```python
from build123d import *

# Parameters (mm, degrees)
F1_R     = 1.5
F1_R_2   = 4
F2_DEPTH = 37.5
F3_DEPTH = 3
F4_DEPTH = 10


with BuildPart() as f2:
    # F1 (on Front) → F2 (new body)
    with BuildSketch(Plane.XZ):
        with BuildLine():
            ThreePointArc((100, 102), (100.585786, 100.585786), (102, 100))
            Line((102, 100), (139, 100))
            ThreePointArc((139, 100), (140.414214, 100.585786), (141, 102))
            Line((141, 102), (141, 139))
            ThreePointArc((141, 139), (140.414214, 140.414214), (139, 141))
            Line((139, 141), (102, 141))
            ThreePointArc((102, 141), (100.585786, 140.414214), (100, 139))
            Line((100, 139), (100, 102))
        make_face()
        with Locations((104.75, 104.75)):
            Circle(F1_R, mode=Mode.SUBTRACT)
        with Locations((136.25, 104.75)):
            Circle(F1_R, mode=Mode.SUBTRACT)
        with Locations((104.75, 136.25)):
            Circle(F1_R, mode=Mode.SUBTRACT)
        with Locations((120.5, 120.5)):
            Circle(F1_R_2, mode=Mode.SUBTRACT)
        with Locations((136.25, 136.25)):
            Circle(F1_R, mode=Mode.SUBTRACT)
        with Locations((104.75, 136.25)):
            Circle(F1_R)
        with Locations((136.25, 136.25)):
            Circle(F1_R)
        with Locations((120.5, 120.5)):
            Circle(F1_R_2)
        with Locations((136.25, 104.75)):
            Circle(F1_R)
        with Locations((104.75, 104.75)):
            Circle(F1_R)
    extrude(amount=F2_DEPTH)

    # F1 (on Front) → F3 (cut)
    with BuildSketch(Plane.XZ):
        with Locations((136.25, 104.75)):
            Circle(F1_R)
        with Locations((104.75, 104.75)):
            Circle(F1_R)
        with Locations((136.25, 136.25)):
            Circle(F1_R)
        with Locations((104.75, 136.25)):
            Circle(F1_R)
    extrude(amount=F3_DEPTH, mode=Mode.SUBTRACT)

    # F1 (on Front) → F4 (join)
    with BuildSketch(Plane.XZ):
        with Locations((120.5, 120.5)):
            Circle(F1_R_2)
    extrude(amount=-F4_DEPTH)


solid = f2.part
```
Geometry check sheet. Reference: the model listing, model coordinates, mm. A direction names the side the tool comes from. Coordinates: 2 decimals unless noted, no trailing zeros. Order: outer loops, then holes, each group sorted by start corner. A loop starts at its lowest first (then second) coordinate and runs counter-clockwise, first axis right, second up. Notation, with made-up numbers: M 76,43.5 L 114,43.5 A9 cw 114,56.5 Z; hole C 70,-5.75 d11. An arc over 180 degrees is marked long. Answer as a JSON object with one key per item and string values.
Q1. Tool access check on faces 1 (the cylindrical face through (104.555, -1.479, 137.737)), 2 (the flat face through (141, -18, 120)). Record the directions out of +Z, -Z, +X, -X, +Y, -Y that give a thin tool (end or side, any length) a straight path to the whole face; none if there is none.
Results are:
{"face 1": "+Y", "face 2": "+Z, -Z, +X, +Y, -Y"}
Q2. Cross-section at C-C on x = 120.5. Record the cut outline in (y, z), and give its area (3 significant figures).
Results are:
{"outline": "M -37.5,100 L 0,100 L 0,116.5 L 10,116.5 L 10,124.5 L 0,124.5 L 0,141 L -37.5,141 Z", "area": "1,620 mm²"}
Q3. Cross-section at D-D on y = 4. Record the cut outline in (x, z), and give its area (3 significant figures).
Results are:
{"outline": "C 120.5,120.5 d8", "area": "50.3 mm²"}
Q4. Release check for a two-part mould opening along Z. For faces 3 (the cylindrical face through (104.555, -1.479, 106.237)), 4 (the cylindrical face through (140.43, -18.49, 140.4)), 5 (the flat face through (105, -3, 136)), 6 (the flat face through (120, -37.5, 121)) record: released by +Z, released by -Z, zero draft, split by the parting line, or undercut.
Results are:
{"face 3": "undercut", "face 4": "released by +Z", "face 5": "undercut", "face 6": "zero draft"}
Q5. Cross-section at B-B on x = 104.75. Record the cut outline in (y, z).
Results are:
{"outline": "M -37.5,100 L 0,100 L 0,103.25 L -3,103.25 L -3,106.25 L 0,106.25 L 0,134.75 L -3,134.75 L -3,137.75 L 0,137.75 L 0,141 L -37.5,141 Z"}
Q6. Depth check by flat-ended pin: pin 1 Ø0.9 at (x, z) = (104.5, 136) entering from +Y; pin 2 Ø4 at (x, z) = (123.5, 108) entering from +Y; pin 3 Ø6 at (y, z) = (3.5, 116.5) entering from -X. Enter the tip coordinate at first touch or a pass-through.
Results are:
{"pin 1": "stops at y = -3", "pin 2": "stops at y = 0", "pin 3": "stops at x = 116.63"}
Q7. Cross-section at A-A on z = 136.25. Record the cut outline in (x, y), and give its area (3 significant figures).
Results are:
{"outline": "M 100,-37.5 L 141,-37.5 L 141,0 L 137.75,0 L 137.75,-3 L 134.75,-3 L 134.75,0 L 106.25,0 L 106.25,-3 L 103.25,-3 L 103.25,0 L 100,0 Z", "area": "1,520 mm²"}
Q8. Scan lines: line 1 (X direction, y = -1.05, z = 136.25); line 2 (Z direction, x = 104, y = -1). Record each from-to range of solid material in increasing order.
Results are:
{"line 1": "x = 100 to 103.25, 106.25 to 134.75, 137.75 to 141", "line 2": "z = 100 to 103.45, 106.05 to 134.95, 137.55 to 141"}
